Design review of the part built by this model. Coordinates are the model's own, in mm. Coordinates: 2 decimals unless noted, no trailing zeros. Loops run counter-clockwise (first coordinate to the right, second up) from the corner with the lowest first, then second, coordinate; pieces in that order, holes last. Notation, with made-up numbers: M 60.25,-38.5 L 98.25,-38.5 A20 cw 98.25,-6.5 Z; hole C -11.5,7.25 d7. An arc over 180 degrees is marked long. Write item = value, one per line. Start each with the question number.
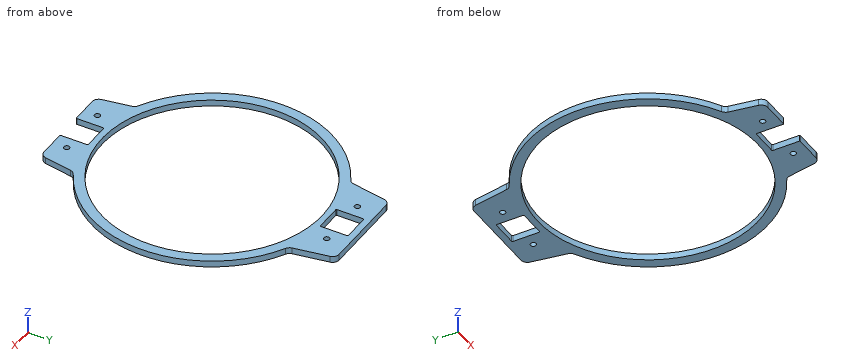
```python
from build123d import *

# Parameters (mm, degrees)
SKETCH2_R           = 83.05
SKETCH2_R_2         = 2.75
BOSS_EXTRUDE1_DEPTH = 4.7498
SKETCH3_R           = 2.75
SKETCH3_R_2         = 2.1
BOSS_EXTRUDE2_DEPTH = 4.7498


with BuildPart() as part:
    # Sketch2 → Boss-Extrude1 (new body)
    with BuildSketch(Plane(origin=(0, 0, 109.855), x_dir=(-1, 0, 0), z_dir=(0, 0, -1))):
        with BuildLine():
            Line((-31.381634904, -108.55), (-11, -108.55))
            ThreePointArc((-11, -108.55), (-10.646446609, -108.403553391), (-10.5, -108.05))
            Line((-10.5, -108.05), (-10.5, -88.05))
            ThreePointArc((-10.5, -88.05), (-10.353553391, -87.696446609), (-10, -87.55))
            Line((-10, -87.55), (10, -87.55))
            ThreePointArc((10, -87.55), (10.353553391, -87.696446609), (10.5, -88.05))
            Line((10.5, -88.05), (10.5, -108.05))
            ThreePointArc((10.5, -108.05), (10.646446609, -108.403553391), (11, -108.55))
            Line((11, -108.55), (31.381634904, -108.55))
            ThreePointArc((31.381634904, -108.55), (34.595572952, -107.380222216), (36.305673669, -104.418240888))
            Line((36.305673669, -104.418240888), (39.974409604, -83.611805478))
            ThreePointArc((39.974409604, -83.611805478), (40.853639928, -81.540739531), (42.55192133, -80.064866772))
            ThreePointArc((42.55192133, -80.064866772), (90.67, 0), (42.55192133, 80.064866772))
            ThreePointArc((42.55192133, 80.064866772), (40.853639928, 81.540739531), (39.974409604, 83.611805478))
            Line((39.974409604, 83.611805478), (35.424038765, 109.418240888))
            ThreePointArc((35.424038765, 109.418240888), (33.713938048, 112.380222216), (30.5, 113.55))
            Line((30.5, 113.55), (-30.5, 113.55))
            ThreePointArc((-30.5, 113.55), (-33.713938048, 112.380222216), (-35.424038765, 109.418240888))
            Line((-35.424038765, 109.418240888), (-39.974409604, 83.611805478))
            ThreePointArc((-39.974409604, 83.611805478), (-40.853639928, 81.540739531), (-42.55192133, 80.064866772))
            ThreePointArc((-42.55192133, 80.064866772), (-90.67, 0), (-42.55192133, -80.064866772))
            ThreePointArc((-42.55192133, -80.064866772), (-40.853639928, -81.540739531), (-39.974409604, -83.611805478))
            Line((-39.974409604, -83.611805478), (-36.305673669, -104.418240888))
            ThreePointArc((-36.305673669, -104.418240888), (-34.595572952, -107.380222216), (-31.381634904, -108.55))
        make_face()
        Circle(SKETCH2_R, mode=Mode.SUBTRACT)
        with Locations((20, 98.05)):
            Circle(SKETCH2_R_2, mode=Mode.SUBTRACT)
        with Locations((-20, 98.05)):
            Circle(SKETCH2_R_2, mode=Mode.SUBTRACT)
        with Locations((20, -98.05)):
            Circle(SKETCH2_R_2, mode=Mode.SUBTRACT)
        with Locations((-20, -98.05)):
            Circle(SKETCH2_R_2, mode=Mode.SUBTRACT)
        with BuildLine():
            Line((10, 87.55), (-10, 87.55))
            ThreePointArc((-10, 87.55), (-10.353553391, 87.696446609), (-10.5, 88.05))
            Line((-10.5, 88.05), (-10.5, 108.05))
            ThreePointArc((-10.5, 108.05), (-10.353553391, 108.403553391), (-10, 108.55))
            Line((-10, 108.55), (10, 108.55))
            ThreePointArc((10, 108.55), (10.353553391, 108.403553391), (10.5, 108.05))
            Line((10.5, 108.05), (10.5, 88.05))
            ThreePointArc((10.5, 88.05), (10.353553391, 87.696446609), (10, 87.55))
        make_face(mode=Mode.SUBTRACT)
    extrude(amount=BOSS_EXTRUDE1_DEPTH)

    # Sketch3 → Boss-Extrude2 (add)
    # profile 1 of 4: a face of its own
    with BuildSketch(Plane.XY.offset(109.855)):
        with Locations((-20, 98.05)):
            Circle(SKETCH3_R)
        with Locations((-20, 98.05)):
            Circle(SKETCH3_R_2, mode=Mode.SUBTRACT)
    # profile 2 of 4: a face of its own
    with BuildSketch(Plane.XY.offset(109.855)):
        with Locations((20, 98.05)):
            Circle(SKETCH3_R)
        with Locations((20, 98.05)):
            Circle(SKETCH3_R_2, mode=Mode.SUBTRACT)
    # profile 3 of 4: a face of its own
    with BuildSketch(Plane.XY.offset(109.855)):
        with Locations((20, -98.05)):
            Circle(SKETCH3_R)
        with Locations((20, -98.05)):
            Circle(SKETCH3_R_2, mode=Mode.SUBTRACT)
    # profile 4 of 4: a face of its own
    with BuildSketch(Plane.XY.offset(109.855)):
        with Locations((-20, -98.05)):
            Circle(SKETCH3_R)
        with Locations((-20, -98.05)):
            Circle(SKETCH3_R_2, mode=Mode.SUBTRACT)
    extrude(amount=-BOSS_EXTRUDE2_DEPTH)


solid = part.part
```
(1) To check wall thickness, follow L1, parallel to Y at x = 0, z = 108.15; L2, parallel to Y at x = -20, z = 106.2; L3, parallel to X at y = -0.5, z = 107.7. State the ranges of each line that lie inside material, in increasing order.
(2) Take a section at C-C (x = 74). State the section outline as (y, z) points (3 decimals), plus the area to 3 significant figures.
(3) Take a section at D-D (z = 107.6). Give the number of separate pieces and of enclosed holes in the cut face, plus the area to 3 significant figures.
(4) Take a section at A-A (x = 0). State the section outline as (y, z) points (3 decimals), plus the area to 3 significant figures.
(5) Take a section at B-B (y = 0). State the section outline as (x, z) points (3 decimals), plus the area to 3 significant figures.
(6) Insertion check: pin 1 (2.5 mm diameter, centred on y = 99.5, z = 108, fed in from -X); pin 2 (2.5 mm diameter, centred on y = -96, z = 107, fed in from -X); pin 3 (2.5 mm diameter, centred on x = 20, y = 98.05, fed in from +Z); pin 4 (2 mm diameter, centred on y = 31, z = 107, fed in from -X). Each pin has a flat end and moves straight along its axis. Give the tip position at first contact, or say it passes through.
Results list:
q1.L1 = -87.55 to -83.05, 83.05 to 87.55, 108.55 to 113.55
q1.L2 = -108.55 to -100.15, -95.95 to -80.61, 80.61 to 95.95, 100.15 to 113.55
q1.L3 = -90.67 to -83.05, 83.05 to 90.67
q2.outline = M -52.393,105.105 L -37.7,105.105 L -37.7,109.855 L -52.393,109.855 Z; M 37.7,105.105 L 52.393,105.105 L 52.393,109.855 L 37.7,109.855 Z
q2.area = 140 mm^2
q3.separate_pieces = 1
q3.enclosed_holes = 6
q3.area = 6,690 mm^2
q4.outline = M -87.55,105.105 L -83.05,105.105 L -83.05,109.855 L -87.55,109.855 Z; M 83.05,105.105 L 87.55,105.105 L 87.55,109.855 L 83.05,109.855 Z; M 108.55,105.105 L 113.55,105.105 L 113.55,109.855 L 108.55,109.855 Z
q4.area = 66.5 mm^2
q5.outline = M -90.67,105.105 L -83.05,105.105 L -83.05,109.855 L -90.67,109.855 Z; M 83.05,105.105 L 90.67,105.105 L 90.67,109.855 L 83.05,109.855 Z
q5.area = 72.4 mm^2
q6.pin_1 = -37.39
q6.pin_2 = -38.01
q6.pin_3 = through
q6.pin_4 = -85.56
